Input: part model. Units: mm. Frame: model coordinates. A direction names the side the tool comes from. Give positions to 0.01 mm unless a question says otherwise; leave off trailing zeros. Write each loop counter-clockwise with the first axis right and the second up, starting at its lowest first coordinate (ties: lowest second). Pieces come first, ordered by that corner, then holes. Notation, with made-up numbers: (39, -21) -> (69, -21) arc R25 cw to (69, 15) -> close; hole circle Ø11 at (7, 0). An arc over 180 degrees is marked (long way). Return JSON: item names as keys, results as strings. Group by question number.
Item 1: Section B-B, the plane z = -67.5. Return loops of the section in (x, y), then the cut area to 3 significant figures.
Item 2: Mould query, pull axis Y, two halves, no side actions, for faces 1 (the face through (49, 0, -68)), 2 (the face through (53, 65, -68)), 3 (the face through (100, 5, -67)). Classes: released by +Y, released by -Y, zero draft, split by the parting line, or undercut.
Item 3: Set-up query: faces 4 (the face through (49, 5, -135)), 5 (the face through (45.63, 69.93, -73.375)), 6 (the face through (54.37, 69.93, -61.625)), 7 (the face through (4.249, 37.115, -7.385)). Return all of +Z, -Z, +X, -X, +Y, -Y with unobstructed straight access to the full face (end or side cutting, diameter ignored); none if empty.
Item 4: Section C-C, the plane z = -103.5. Return loops of the section in (x, y), then the cut area to 3 significant figures.
Item 5: Section D-D, the plane x = 57.5. Return loops of the section in (y, z), then the cut area to 3 significant figures.
Item 6: Section A-A, the plane y = 70. Return loops of the section in (x, z).
Item 7: Pin query (flat end, axial travel): P1, Ø10, axis at y = 33, z = -17, coming from the +X side; P2, Ø8, axis at x = 19.5, z = -80.5, coming from the +Y side; P3, Ø10, axis at x = 83.5, z = -101, coming from the +Y side. Return the tip coordinate at first contact, or that it passes through.
Item 8: Line query: line 1 (Y direction, x = 50, z = -67.5); line 2 (Y direction, x = 62.5, z = -95); line 3 (Y direction, x = 46, z = -67). Output: solid intervals per line, ascending. Write a range as [from, to].
from build123d import *

# Parameters (mm, degrees)
SKETCH1_W                    = 100
SKETCH1_H                    = 135
BOTTOMPLATE_DEPTH            = 10
SKETCH2_R                    = 2.5
TOPPLATFORMSUPPORT_DEPTH     = 55
TOPTHREADEDRODPLATFORM_DEPTH = 10
CUT_EXTRUDE2_REACH           = 185.984
SKETCH5_R                    = 2.5


with BuildPart() as part:
    # Sketch1 → BottomPlate (new body)
    with BuildSketch(Plane(origin=(0, 0, 0), x_dir=(1, 0, 0), z_dir=(0, 1, 0))):
        with Locations((50, 67.5)):
            Rectangle(SKETCH1_W, SKETCH1_H)
    extrude(amount=BOTTOMPLATE_DEPTH)

    # Sketch2 → TopPlatformSupport (add)
    with BuildSketch(Plane(origin=(0, 10, 0), x_dir=(1, 0, 0), z_dir=(0, 1, 0))):
        with Locations(Location((95, 130, 0), (0, 0, 90))):
            Circle(SKETCH2_R)
        with Locations(Location((5, 5, 0), (0, 0, 90))):
            Circle(SKETCH2_R)
    extrude(amount=TOPPLATFORMSUPPORT_DEPTH)

    # Sketch3 → TopThreadedRodPlatform (add)
    with BuildSketch(Plane(origin=(0, 65, 0), x_dir=(1, 0, 0), z_dir=(0, 1, 0))):
        Polygon((90, 135), (0, 10), (0, 0), (10, 0), (100, 125), (100, 135), align=None)
    extrude(amount=TOPTHREADEDRODPLATFORM_DEPTH)

    # Cut-Extrude2: up to this plane
    cut_extrude2_end = Plane(origin=(90, 75, -135), z_dir=(0.8115343414514944, 0, 0.584304725845076))
    # Sketch5 → Cut-Extrude2 (cut, up to the surface)
    with BuildSketch(Plane(origin=(100, 0, 0), x_dir=(0, 0, -1), z_dir=(1, 0, 0)), mode=Mode.PRIVATE) as cut_extrude2_sk1:
        with Locations((67.5, 70)):
            Circle(SKETCH5_R)
    cut_extrude2_tool1 = split(extrude(cut_extrude2_sk1.sketch, amount=-CUT_EXTRUDE2_REACH, mode=Mode.PRIVATE), bisect_by=cut_extrude2_end, keep=Keep.BOTH, mode=Mode.PRIVATE)
    add(cut_extrude2_tool1.solids().sort_by_distance((100, 70, -67.5))[0], mode=Mode.SUBTRACT)


solid = part.part
Answer below:
{
 "1": {"outline": "(0, 0) -> (100, 0) -> (100, 10) -> (0, 10) -> close; (41.4, 65) -> (58.6, 65) -> (58.6, 67.5) -> (41.4, 67.5) -> close; (41.4, 72.5) -> (58.6, 72.5) -> (58.6, 75) -> (41.4, 75) -> close", "area": "1,090 mm2"},
 "2": {"face 1": "released by -Y", "face 2": "undercut", "face 3": "zero draft"},
 "3": {"face 4": "-Z, +X, -X, +Y, -Y", "face 5": "-Z, -X, +Y", "face 6": "+Z, +X, +Y", "face 7": "none"},
 "4": {"outline": "(0, 0) -> (100, 0) -> (100, 10) -> (0, 10) -> close; (67.32, 65) -> (84.52, 65) -> (84.52, 75) -> (67.32, 75) -> close", "area": "1,170 mm2"},
 "5": {"outline": "(0, -135) -> (10, -135) -> (10, 0) -> (0, 0) -> close; (65, -89.86) -> (75, -89.86) -> (75, -65.97) -> (71.98, -65.97) arc R2.5 cw (long way) to (68.02, -65.97) -> (65, -65.97) -> close", "area": "1,570 mm2"},
 "6": {"outline": "(0, -10) -> (39.6, -65) -> (56.8, -65) -> (10, 0) -> (0, 0) -> close; (43.2, -70) -> (90, -135) -> (100, -135) -> (100, -125) -> (60.4, -70) -> close"},
 "7": {"P1": "passes through", "P2": "stops at y = 10", "P3": "stops at y = 75"},
 "8": {"line 1": "y = [0, 10], [65, 67.5], [72.5, 75]", "line 2": "y = [0, 10], [65, 75]", "line 3": "y = [0, 10], [65, 67.55], [72.45, 75]"}
}
